Part print with two shaded views. Sizes in mm from the minimum x, y, z corner. Coordinates: 2 decimals unless noted, no trailing zeros. Write each loop counter-clockwise with the first axis right and the second up, starting at its lowest first coordinate (ties: lowest second). Pieces come first, ordered by that corner, then holes.
Q1. Band-saw the part on D-D, the plane x = 11.5. Write the cut outline in (y, z).
Q2. Drill centre lines: probe 1 along X at (y, z) = (13.75, 1.35); probe 2 along X at (y, z) = (13.5, 1.1) (1 decimal); probe 3 along Y at (x, z) = (5, 2.3). Where is each one in solid material? Low to high.
Q3. Pull direction X, two halves, no side cores. Call the marked faces 1, 2 and 3: released by +X, released by -X, zero draft, split by the parting line, or undercut.
Q4. Band-saw the part on A-A, the plane x = 15. Write the cut outline in (y, z) (1 decimal), plus the area to 3 significant figures.
Q5. Band-saw the part on C-C, the plane z = 1.9. Write the cut outline in (x, y).
Q6. Band-saw the part on B-B, the plane y = 7.75. Write the cut outline in (x, z).
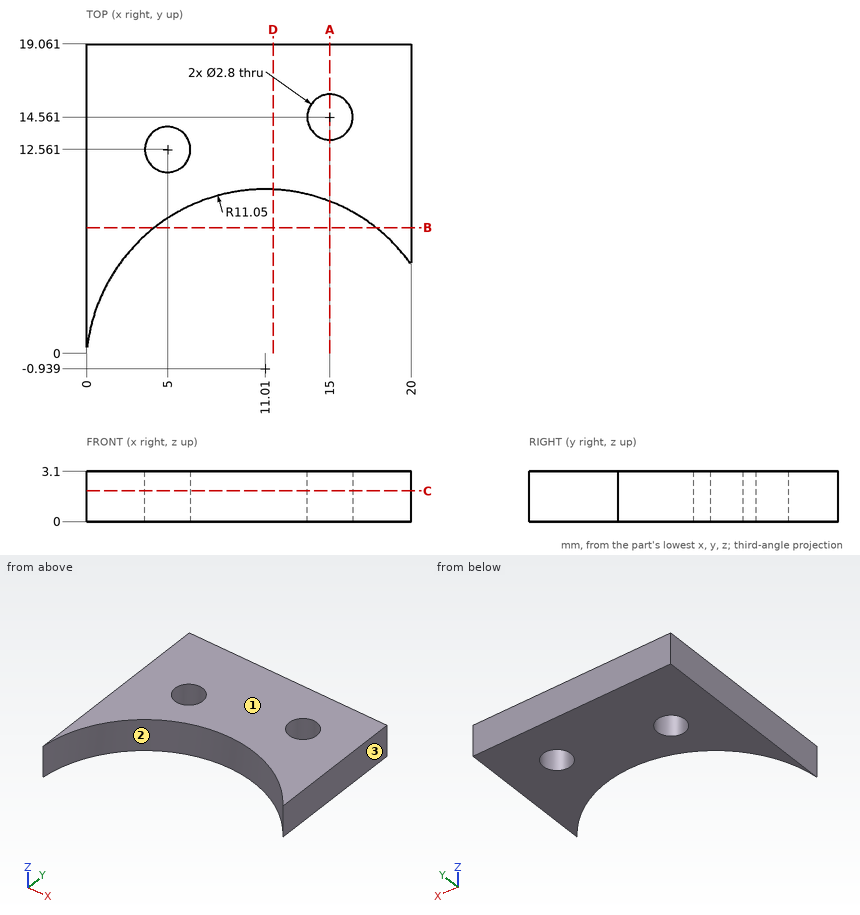
Answer sheet:
1. outline: (10.1, 0) - (19.06, 0) - (19.06, 3.1) - (10.1, 3.1) - close
2. probe 1: x = 0 to 4.26, 5.74 to 13.86, 16.14 to 20
2. probe 2: x = 0 to 4, 6 to 14.1, 15.9 to 20
2. probe 3: y = 8.33 to 11.16, 13.96 to 19.06
3. face 1: zero draft
3. face 2: undercut
3. face 3: released by +X
4. outline: (9.4, 0) - (13.2, 0) - (13.2, 3.1) - (9.4, 3.1) - close; (16, 0) - (19.1, 0) - (19.1, 3.1) - (16, 3.1) - close
4. area: 21.4 mm2
5. outline: (0, 0) arc R11.05 cw to (20, 5.49) - (20, 19.06) - (0, 19.06) - close; hole circle Ø2.8 at (5, 12.56); hole circle Ø2.8 at (15, 14.56)
6. outline: (0, 0) - (4.18, 0) - (4.18, 3.1) - (0, 3.1) - close; (17.84, 0) - (20, 0) - (20, 3.1) - (17.84, 3.1) - close
